Build history of the part. All positions in model axes, mm. A direction names the side the tool comes from. Round coordinates to 2 decimals unless told otherwise and drop trailing zeros. Order: outer loops, then holes, each group sorted by start corner. A loop starts at its lowest first (then second) coordinate and runs counter-clockwise, first axis right, second up. Notation, with made-up numbers: M 20,-38 L 73,-38 A7 cw 73,-27 Z; hole C 66.5,72.25 d10. An arc over 180 degrees is marked long. Use CSV: the item, a comma, the result in double quotes.
Autodesk Inventor part; units mm, degrees
ref_plane "Work Plane3" through (-2.6427, -2.7179, 0) normal (0, 1, 0) x (0, 0, 1)
ref_plane "YZ Plane" through (0, 0, 0) normal (1, 0, 0) x (0, 1, 0)
ref_plane "XZ Plane" through (0, 0, 0) normal (0, 1, 0) x (-1, 0, 0)
ref_plane "Work Plane1" through (0, 0, 0) normal (0, 0, 1) x (1, 0, 0)
sketch "Sketch1" plane through (0, 0, 0) normal (0, 0, 1) x (1, 0, 0)
  circle A0 centre (2.6061, 6.2821) radius 1.5 construction
  circle A1 centre (22.6061, 6.2821) radius 1.5 construction
  line L0 (-2.6427, 15.6321) -> (-2.6427, -2.7179) construction
  line L1 (-2.6427, -2.7179) -> (30.1061, -2.7179) construction
  line L2 (30.1061, -2.7179) -> (30.1061, -39.6443) construction
  line L3 (30.1061, -39.6443) -> (66.9651, 7.5331) construction
  line L4 (66.9651, 7.5331) -> (66.9651, 15.6321) construction
  line L5 (66.9651, 15.6321) -> (-2.6427, 15.6321) construction
  circle A2 centre (12.3511, 11.6321) radius 1.45 construction
  circle A3 centre (41.9344, -5.4679) radius 1.45 construction
  circle A4 centre (34.1061, -5.4679) radius 1.45 construction
  circle A5 centre (54.6178, 11.6321) radius 1.45 construction
  circle A6 centre (-0.6427, 11.6823) radius 1.45 construction
  circle A7 centre (29.5857, 11.6321) radius 1.45 construction
  circle A8 centre (51.7579, -5.4342) radius 1.45 construction
  circle A9 centre (34.1061, -24.4536) radius 1.45 construction
  circle A10 centre (47.169, 11.6321) radius 1.45 construction
  line L6 (-2.0689, 15.0821) -> (-2.0689, 2.6821) construction
  line L7 (27.2811, 15.0821) -> (27.2811, 2.6821) construction
  line L8 (32.1612, -8.9378) -> (42.8353, -8.9378)
  line L9 (42.8353, -8.9378) -> (51.0915, -0.6816)
  line L10 (51.0915, -0.6816) -> (51.0915, 15.6321)
  line L11 (32.1612, -8.9378) -> (32.1612, 15.6321)
  line L12 (32.1612, 15.6321) -> (51.0915, 15.6321)
  circle A11 centre (34.1061, -5.4679) radius 1.55
  circle A12 centre (41.9344, -5.4679) radius 1.55
  circle A13 centre (47.169, 11.6321) radius 1.55
  line L13 (32.1612, 15.6321) -> (51.0915, 15.6321)
  line L14 (51.0915, 15.6321) -> (51.0915, 20.6321)
  line L15 (51.0915, 20.6321) -> (32.1612, 20.6321)
  line L16 (32.1612, 20.6321) -> (32.1612, 15.6321)
  point P0 (0, 0)
  dimension "d0" = 135
  dimension "d1" = 3.1
  dimension "d2" = 3.1
  dimension "d3" = 3.1
  dimension "d16" = 5
extrude "Extrusion1" add sketch "Sketch1" along normal blind 4
sketch "Sketch5" plane through (32.1612, 20.6321, 0) normal (0, 1, 0) x (1, 0, 0)
  circle A0 centre (-19.5551, -14.65) radius 15.24 construction
  circle A1 centre (-19.3039, -15.5) radius 15.5 construction
  line L0 (-34.8039, 0) -> (-34.8039, -32) construction
  line L1 (34.8039, 0) -> (-34.8039, 0) construction
  line L2 (0, 0) -> (18.9303, 0) construction
  line L3 (0, 0) -> (0, -4) construction
  line L4 (18.9303, -4) -> (0, -4) construction
  line L5 (18.9303, 0) -> (18.9303, -4) construction
  line L6 (0, 0) -> (18.9303, 0) construction
  line L7 (0, 0) -> (-19.3058, 0) construction
  line L8 (0, 0) -> (-19.3039, 0)
  line L9 (-34.8039, -32) -> (0, -32)
  line L10 (0, -32) -> (0, 0)
  arc A2 (-34.8039, -15.5) -> (-19.3039, 0) centre (-19.3039, -15.5) ccw
  line L11 (-34.8039, -32) -> (-34.8039, -15.5)
  point P0 (-32.1612, 0)
  dimension "d21" = 31
ref_plane "Work Plane3" through (-2.6427, -2.7179, 0) normal (0, 1, 0) x (0, 0, 1)
extrude "Extrusion5" add sketch "Sketch5" against normal up to surface (23.35 mm away)
fillet "Fillet1" radius 2 5 edges at (-2.6427, 8.9571, 15.5) (12.8573, 8.9571, 0) (32.1612, 8.9571, 32) (-2.6427, 8.9571, 32) (32.1612, 8.9571, 4)
properties part number "cellSTORM_alviumadapter"
(1) Cut at A-A, the plane x = 27.5. Give the cut face in (y, z), and give its area (3 significant figures).
Answer block:
outline,"M -2.72,0 L 20.63,0 L 20.63,10.42 L -2.72,10.42 Z; M -2.72,20.58 L 20.63,20.58 L 20.63,32 L -2.72,32 Z"
area,"510 mm²"
(2) Cut at D-D, the plane x = 14.5. Give the cut face in (y, z).
Answer block:
outline,"M -2.72,30.91 L 20.63,30.91 L 20.63,32 L -2.72,32 Z"
(3) Tool access for faces 1 (the face through (32.161, -6, 2)), 2 (the face through (32.161, 9, 18)), 3 (the face through (23.56, 9.12, 26.71)): list every direction of +Z, -Z, +X, -X, +Y, -Y with a clear straight run to the whole face (end or side of a thin tool).
Answer block:
face 1,"+Z, -Z, -X, -Y"
face 2,"+Z, +X, +Y, -Y"
face 3,"+Y, -Y"
(4) Wall check: line 1 (Y direction, x = 1.5, z = 26.5); line 2 (X direction, y = 12.25, z = 15.5); line 3 (Z direction, x = 38, y = 3.25). Give the ranges that are in metal, low to high. Write a range as from..to.
Answer block:
line 1,"y = -2.72..20.63"
line 2,"x = 28.36..32.16"
line 3,"z = 0..4"
(5) Drop flat-ended pins along their axis: pin 1 (18.5 mm diameter, centred on x = 12.86, z = 15.5, fed in from -Y); pin 2 (4.5 mm diameter, centred on y = -4.5, z = 1.5, fed in from -X); pin 3 (5.5 mm diameter, centred on x = 46, y = 0, fed in from +Z); pin 4 (12 mm diameter, centred on x = 9.5, y = 13, fed in from -Z). Give the stop position or say it passes through.
Answer block:
pin 1,"passes through"
pin 2,"stops at x = 21.99"
pin 3,"stops at z = 4"
pin 4,"stops at z = 27.86"
(6) Cut at B-B, the plane y = 9.5. Give the cut face in (x, z).
Answer block:
outline,"M -2.64,26.63 A2 ccw 0.9,25.36 A15.5 cw long 22.72,3.54 A2 ccw 23.99,0 L 51.09,0 L 51.09,4 L 34.16,4 A2 cw 32.16,6 L 32.16,30 A2 ccw 30.16,32 L -0.64,32 A2 ccw -2.64,30 Z"
(7) Cut at C-C, the plane z = 15.5. Give the cut face in (x, y), and give its area (3 significant figures).
Answer block:
outline,"M 28.36,-2.72 L 32.16,-2.72 L 32.16,20.63 L 28.36,20.63 Z"
area,"88.8 mm²"
(8) Two-plate mould, pull along X, no slides. Class faces 4 (the face through (-2.643, 9, 28)), 5 (the face through (46.833, 13.145, 1.972)), 6 (the face through (46.906, -4.867, 1.972)), 7 (the face through (35.585, -5.933, 1.972)): released by +X, released by -X, zero draft, split by the parting line, or undercut.
Answer block:
face 4,"released by -X"
face 5,"undercut"
face 6,"released by +X"
face 7,"undercut"
